from build123d import *

# Parameters (mm, degrees)
CYLINDER757_R               = 1.5
CYLINDER757_DEPTH           = 100
CYLINDER757_PLACEMENT_ANGLE = 100
CYLINDER755_R               = 1.5
CYLINDER755_DEPTH           = 100
CYLINDER755_PLACEMENT_ANGLE = 135
CYLINDER759_R               = 1.5
CYLINDER759_DEPTH           = 100
CYLINDER761_R               = 1.5
CYLINDER761_DEPTH           = 100
CYLINDER761_PLACEMENT_ANGLE = 225
CYLINDER754_R               = 1.5
CYLINDER754_DEPTH           = 100
CYLINDER758_R               = 1.5
CYLINDER758_DEPTH           = 100
CYLINDER758_PLACEMENT_ANGLE = 55
CYLINDER756_R               = 1.5
CYLINDER756_DEPTH           = 100
CYLINDER760_R               = 1.5
CYLINDER760_DEPTH           = 100
CYLINDER760_PLACEMENT_ANGLE = 45
TUBE079_R                   = 58
TUBE079_R_2                 = 38
TUBE079_DEPTH               = 1


with BuildPart() as obj1:
    # Cylinder757 → Cylinder757 (new body)
    with BuildSketch(Plane.XY):
        Circle(CYLINDER757_R)
    extrude(amount=CYLINDER757_DEPTH)


with BuildPart() as obj1_1:
    # Cylinder757 placement: moved
    add(obj1.part.moved(Location((41.004432, -9.090464, 0))).rotate(Axis((41.004432, -9.090464, 0), (0, 0, 1)), CYLINDER757_PLACEMENT_ANGLE))


with BuildPart() as obj2:
    # Cylinder755 → Cylinder755 (new body)
    with BuildSketch(Plane.XY):
        Circle(CYLINDER755_R)
    extrude(amount=CYLINDER755_DEPTH)


with BuildPart() as obj2_1:
    # Cylinder755 placement: moved
    add(obj2.part.moved(Location((38.80294, 16.072704, 0))).rotate(Axis((38.80294, 16.072704, 0), (0, 0, 1)), CYLINDER755_PLACEMENT_ANGLE))


with BuildPart() as obj3:
    # Cylinder759 → Cylinder759 (new body)
    with BuildSketch(Plane(origin=(16.072704, 38.80294, 0), x_dir=(-1, 0, 0), z_dir=(0, 0, 1))):
        Circle(CYLINDER759_R)
    extrude(amount=CYLINDER759_DEPTH)


with BuildPart() as obj4:
    # Cylinder761 → Cylinder761 (new body)
    with BuildSketch(Plane.XY):
        Circle(CYLINDER761_R)
    extrude(amount=CYLINDER761_DEPTH)


with BuildPart() as obj4_1:
    # Cylinder761 placement: moved
    add(obj4.part.moved(Location((-16.072704, 38.80294, 0))).rotate(Axis((-16.072704, 38.80294, 0), (0, 0, 1)), CYLINDER761_PLACEMENT_ANGLE))


with BuildPart() as obj5:
    # Cylinder754 → Cylinder754 (new body)
    with BuildSketch(Plane(origin=(-38.80294, 16.072704, 0), x_dir=(0, -1, 0), z_dir=(0, 0, 1))):
        Circle(CYLINDER754_R)
    extrude(amount=CYLINDER754_DEPTH)


with BuildPart() as obj6:
    # Cylinder758 → Cylinder758 (new body)
    with BuildSketch(Plane.XY):
        Circle(CYLINDER758_R)
    extrude(amount=CYLINDER758_DEPTH)


with BuildPart() as obj6_1:
    # Cylinder758 placement: moved
    add(obj6.part.moved(Location((-41.004432, -9.090464, 0))).rotate(Axis((-41.004432, -9.090464, 0), (0, 0, -1)), CYLINDER758_PLACEMENT_ANGLE))


with BuildPart() as obj7:
    # Cylinder756 → Cylinder756 (new body)
    with BuildSketch(Plane(origin=(-16.072704, -38.80294, 0), x_dir=(1, 0, 0), z_dir=(0, 0, 1))):
        Circle(CYLINDER756_R)
    extrude(amount=CYLINDER756_DEPTH)


with BuildPart() as compound709:
    # Cylinder760 → Cylinder760 (new body)
    with BuildSketch(Plane.XY):
        Circle(CYLINDER760_R)
    extrude(amount=CYLINDER760_DEPTH)


with BuildPart() as compound709_1:
    # Cylinder760 placement: moved
    add(compound709.part.moved(Location((16.072704, -38.80294, 0))).rotate(Axis((16.072704, -38.80294, 0), (0, 0, 1)), CYLINDER760_PLACEMENT_ANGLE))

    # Compound709: union obj1, obj2, obj3, obj4, obj5, obj6, obj7
    add(obj1_1.part)
    add(obj2_1.part)
    add(obj3.part)
    add(obj4_1.part)
    add(obj5.part)
    add(obj6_1.part)
    add(obj7.part)


with BuildPart() as obj8:
    # Tube079 → Tube079 (new body)
    with BuildSketch(Plane.XY.offset(42)):
        Circle(TUBE079_R)
        Circle(TUBE079_R_2, mode=Mode.SUBTRACT)
    extrude(amount=TUBE079_DEPTH)

    # Cut325: cut Compound709
    add(compound709_1.part, mode=Mode.SUBTRACT)


solid = obj8.part
Geometry check sheet. Reference: the model listing, model coordinates, mm. Give positions to 0.01 mm unless a question says otherwise; leave off trailing zeros. Order: outer loops, then holes, each group sorted by start corner. A loop starts at its lowest first (then second) coordinate and runs counter-clockwise, first axis right, second up.
1) Cross-section at D-D (x = -46.5). Record the boundary of the cut face in (y, z), then the cut area to 3 significant figures.
Results are:
outline: (-34.67, 42) - (34.67, 42) - (34.67, 43) - (-34.67, 43) - close
area: 69.3 mm2
2) Cross-section at B-B (x = 2.5). Record the boundary of the cut face in (y, z), then the cut area to 3 significant figures.
Results are:
outline: (-57.95, 42) - (-37.92, 42) - (-37.92, 43) - (-57.95, 43) - close; (37.92, 42) - (57.95, 42) - (57.95, 43) - (37.92, 43) - close
area: 40.1 mm2
3) Draft check along X on faces 1 (the cylindrical face through (26.76, -51.46, 42.49)), 2 (the flat face through (12, -38, 43)), 3 (the cylindrical face through (-37.538, 15.266, 42.493)). Enter one of: released by +X, released by -X, zero draft, split by the parting line, or undercut.
Results are:
face 1: split by the parting line
face 2: zero draft
face 3: undercut
4) Material ranges on probe 1 along Y at (x, z) = (-1.5, 42.2); probe 2 along X at (y, z) = (1, 42.45); probe 3 along X at (y, z) = (-10, 42.8), recorded low to high.
Results are:
probe 1: y = -57.98 to -37.97, 37.97 to 57.98
probe 2: x = -57.99 to -37.99, 37.99 to 57.99
probe 3: x = -57.13 to -42.2, -39.81 to -36.66, 36.66 to 39.81, 42.2 to 57.13
5) Cross-section at C-C (z = 42.2). Give the number of separate pieces and of enclosed holes in the cut face, then the cut area to 3 significant figures.
Results are:
separate pieces: 1
enclosed holes: 9
area: 5,980 mm2
6) Cross-section at A-A (y = 0). Record the boundary of the cut face in (x, z), then the cut area to 3 significant figures.
Results are:
outline: (-58, 42) - (-38, 42) - (-38, 43) - (-58, 43) - close; (38, 42) - (58, 42) - (58, 43) - (38, 43) - close
area: 40.0 mm2
